```python
from build123d import *

# Parameters (mm, degrees)
SKETCH1_W           = 42
SKETCH1_H           = 33
BOSS_EXTRUDE1_DEPTH = 5
SKETCH2_W           = 33
SKETCH2_H           = 5
BOSS_EXTRUDE2_DEPTH = 60
SKETCH3_W           = 33
SKETCH3_H           = 5
BOSS_EXTRUDE3_DEPTH = 52
FILLET1_R           = 5
SKETCH6_R           = 1.933769561
SKETCH6_R_2         = 1.936009006
CUT_EXTRUDE1_DEPTH  = 55
SKETCH7_R           = 3.5
SKETCH7_R_2         = 1.65
SKETCH7_R_3         = 3.75
CUT_EXTRUDE6_DEPTH  = 3
SKETCH8_R           = 1.65
CUT_EXTRUDE7_DEPTH  = 9
CUT_EXTRUDE8_DEPTH  = 3


with BuildPart() as part:
    # Sketch1 → Boss-Extrude1 (new body)
    with BuildSketch(Plane(origin=(0, 0, 0), x_dir=(1, 0, 0), z_dir=(0, 1, 0))):
        with Locations((21, 16.5)):
            Rectangle(SKETCH1_W, SKETCH1_H)
    extrude(amount=BOSS_EXTRUDE1_DEPTH)

    # Sketch2 → Boss-Extrude2 (add)
    with BuildSketch(Plane.ZY):
        with Locations((-16.5, 2.5)):
            Rectangle(SKETCH2_W, SKETCH2_H)
    extrude(amount=BOSS_EXTRUDE2_DEPTH)

    # Sketch3 → Boss-Extrude3 (add)
    with BuildSketch(Plane(origin=(42, 0, 0), x_dir=(0, 0, -1), z_dir=(1, 0, 0))):
        with Locations((16.5, 2.5)):
            Rectangle(SKETCH3_W, SKETCH3_H)
    extrude(amount=BOSS_EXTRUDE3_DEPTH)

    # Fillet1
    fillet1_edges = [part.edges().sort_by_distance(p)[0] for p in [
        (-60, 2.5, 0),
        (-60, 2.5, -33),
        (94, 2.5, 0),
        (94, 2.5, -33),
    ]]
    fillet(fillet1_edges, radius=FILLET1_R)

    # Sketch6 → Cut-Extrude1 (cut)
    with BuildSketch(Plane(origin=(0, 5, 0), x_dir=(1, 0, 0), z_dir=(0, 1, 0))):
        with Locations(Location((-53.892928071, 16.206648626, 0), (0, 0, 270))):
            Circle(SKETCH6_R)
        with BuildLine():
            Line((-33.231112903, 14.928003086), (-32.804010339, 15.222003341))
            ThreePointArc((-32.804010339, 15.222003341), (-32.373392107, 17.150567334), (-34.01401443, 18.251998007))
            ThreePointArc((-34.01401443, 18.251998007), (-35.37580525, 17.583221312), (-35.704007275, 16.101998866))
            ThreePointArc((-35.704007275, 16.101998866), (-34.750203351, 14.919643697), (-33.231112903, 14.928003086))
        make_face()
        with BuildLine():
            ThreePointArc((64.846014701, 15.211997211), (66.795875027, 14.926365069), (67.776015126, 16.636004329))
            ThreePointArc((67.776015126, 16.636004329), (66.782491719, 18.081747119), (65.034015201, 17.940004945))
            ThreePointArc((65.034015201, 17.940004945), (64.284233669, 16.621194208), (64.846014701, 15.211997211))
        make_face()
        with Locations(Location((86.291564463, 16.259906017, 0), (0, 0, 270))):
            Circle(SKETCH6_R_2)
    extrude(amount=-CUT_EXTRUDE1_DEPTH, mode=Mode.SUBTRACT)

    # Sketch7 → Cut-Extrude6 (cut)
    # profile 1 of 4: a face of its own
    with BuildSketch(Plane(origin=(0, 5, 0), x_dir=(1, 0, 0), z_dir=(0, 1, 0))):
        with Locations(Location((3.750000566, 28.5, 0), (0, 0, 270))):
            Circle(SKETCH7_R)
        with Locations(Location((3.750000566, 28.5, 0), (0, 0, 270))):
            Circle(SKETCH7_R_2, mode=Mode.SUBTRACT)
    # profile 2 of 4: a face of its own
    with BuildSketch(Plane(origin=(0, 5, 0), x_dir=(1, 0, 0), z_dir=(0, 1, 0))):
        with Locations(Location((3.750000566, 4.500000179, 0), (0, 0, 270))):
            Circle(SKETCH7_R)
        with Locations(Location((3.750000566, 4.500000179, 0), (0, 0, 270))):
            Circle(SKETCH7_R_2, mode=Mode.SUBTRACT)
    # profile 3 of 4: a face of its own
    with BuildSketch(Plane(origin=(0, 5, 0), x_dir=(1, 0, 0), z_dir=(0, 1, 0))):
        with Locations((38.25, 3.500000179)):
            Circle(SKETCH7_R_3)
        with Locations(Location((38.25, 3.500000179, 0), (0, 0, 270))):
            Circle(SKETCH7_R_2, mode=Mode.SUBTRACT)
    # profile 4 of 4: a face of its own
    with BuildSketch(Plane(origin=(0, 5, 0), x_dir=(1, 0, 0), z_dir=(0, 1, 0))):
        with Locations((38.25, 29.5)):
            Circle(SKETCH7_R_3)
        with Locations(Location((38.25, 29.5, 0), (0, 0, 270))):
            Circle(SKETCH7_R_2, mode=Mode.SUBTRACT)
    extrude(amount=-CUT_EXTRUDE6_DEPTH, mode=Mode.SUBTRACT)

    # Sketch8 → Cut-Extrude7 (cut)
    with BuildSketch(Plane(origin=(0, 5, 0), x_dir=(1, 0, 0), z_dir=(0, 1, 0))):
        with Locations(Location((38.25, 3.500000179, 0), (0, 0, 270))):
            Circle(SKETCH8_R)
        with Locations(Location((3.750000566, 28.5, 0), (0, 0, 270))):
            Circle(SKETCH8_R)
        with Locations(Location((3.750000566, 4.500000179, 0), (0, 0, 270))):
            Circle(SKETCH8_R)
        with Locations(Location((38.25, 29.5, 0), (0, 0, 270))):
            Circle(SKETCH8_R)
    extrude(amount=-CUT_EXTRUDE7_DEPTH, mode=Mode.SUBTRACT)

    # Sketch9 → Cut-Extrude8 (cut)
    with BuildSketch(Plane.XZ):
        Polygon((-50.602031537, -16.206648626), (-52.247479804, -13.356648626), (-55.538376338, -13.356648626), (-57.183824606, -16.206648626), (-55.538376338, -19.056648626), (-52.247479804, -19.056648626), align=None)
        Polygon((-30.708442047, -16.501258638), (-32.353890314, -13.651258638), (-35.644786848, -13.651258638), (-37.290235116, -16.501258638), (-35.644786848, -19.351258638), (-32.353890314, -19.351258638), align=None)
        Polygon((69.321562817, -16.500838902), (67.67611455, -13.650838902), (64.385218016, -13.650838902), (62.739769748, -16.500838902), (64.385218016, -19.350838902), (67.67611455, -19.350838902), align=None)
        Polygon((89.582460998, -16.259906017), (87.93701273, -13.409906017), (84.646116196, -13.409906017), (83.000667929, -16.259906017), (84.646116196, -19.109906017), (87.93701273, -19.109906017), align=None)
    extrude(amount=-CUT_EXTRUDE8_DEPTH, mode=Mode.SUBTRACT)


solid = part.part
```
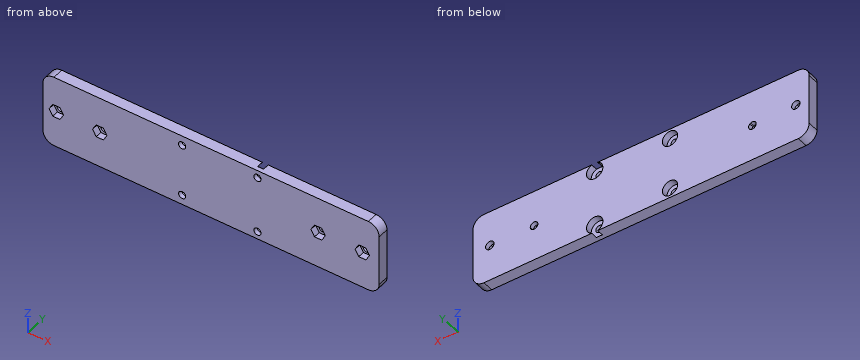
Part model, mm, in its own coordinate system. Round coordinates to 2 decimals unless told otherwise and drop trailing zeros. Loops run counter-clockwise (first coordinate to the right, second up) from the corner with the lowest first, then second, coordinate; pieces in that order, holes last.
1. Slice it at A-A (x = 3.75). Give the cut face in (y, z).
Solutions:
outline: (0, -33) - (5, -33) - (5, -32) - (2, -32) - (2, -30.15) - (0, -30.15) - close; (0, -26.85) - (2, -26.85) - (2, -25) - (5, -25) - (5, -8) - (2, -8) - (2, -6.15) - (0, -6.15) - close; (0, -2.85) - (2, -2.85) - (2, -1) - (5, -1) - (5, 0) - (0, 0) - close
2. Drill centre lines: line 1 along X through (y, z) = (2.85, -27); line 2 along X through (y, z) = (2.45, -28.5); line 3 along Z through (x, y) = (85, 0.45). Where is each one in solid material? Low to high.
Solutions:
line 1: x = -60 to 0.59, 6.91 to 35.45, 41.05 to 94
line 2: x = -59.97 to 0.25, 7.25 to 34.64, 41.86 to 93.97
line 3: z = -33 to -19.11, -13.41 to 0
3. Slice it at B-B (x = 38.25). Give the cut face in (y, z).
Solutions:
outline: (0, -33) - (2, -33) - (2, -31.15) - (0, -31.15) - close; (0, -27.85) - (2, -27.85) - (2, -25.75) - (5, -25.75) - (5, -7.25) - (2, -7.25) - (2, -5.15) - (0, -5.15) - close; (0, -1.85) - (2, -1.85) - (2, 0) - (0, 0) - close
